Autodesk Inventor part; units mm, degrees
ref_plane "YZ Plane" through (0, 0, 0) normal (1, 0, 0) x (0, 1, 0)
ref_plane "XZ Plane" through (0, 0, 0) normal (0, 1, 0) x (-1, 0, 0)
ref_plane "XY Plane" through (0, 0, 0) normal (0, 0, 1) x (1, 0, 0)
sketch "Sketch1" plane through (0, 0, 0) normal (0, 1, 0) x (-1, 0, 0)
  line L0 (7.4919, 7.8851) -> (-12.5081, 7.8851)
  line L1 (-12.5081, 7.8851) -> (-12.5081, -12.1149)
  line L2 (-12.5081, -12.1149) -> (7.4919, -12.1149)
  line L3 (7.4919, -12.1149) -> (7.4919, 7.8851)
  line L4 (8.4919, 8.8851) -> (-13.5081, 8.8851)
  line L5 (-13.5081, 8.8851) -> (-13.5081, -13.1149)
  line L6 (-13.5081, -13.1149) -> (8.4919, -13.1149)
  line L7 (8.4919, -13.1149) -> (8.4919, 8.8851)
  point P0 (0, 0)
  dimension "d0" = 20
  dimension "d1" = 20
  dimension "d2" = 22
  dimension "d3" = 22
  dimension "d4" = 1
  dimension "d5" = 1
extrude "Extrusion1" add sketch "Sketch1" along normal blind 10 contours L3 L2 L1 L0 | L7 L6 L5 L4
sketch "Sketch2" plane through (0, 0, 0) normal (0, 1, 0) x (-1, 0, 0)
  line L0 (7.4919, 7.8851) -> (-12.5081, 7.8851)
  line L1 (-12.5081, 7.8851) -> (-12.5081, -12.1149)
  line L2 (-12.5081, -12.1149) -> (7.4919, -12.1149)
  line L3 (7.4919, -12.1149) -> (7.4919, 7.8851)
  line L4 (8.4919, -13.1149) -> (8.4919, 8.8851)
  line L5 (8.4919, 8.8851) -> (-13.5081, 8.8851)
  point P0 (0, 0)
  dimension "d8" = 20
  dimension "d9" = 20
  dimension "d10" = 1
  dimension "d11" = 1
extrude "Extrusion2" cut sketch "Sketch2" along normal blind 9
fillet "Fillet1" radius 2 4 edges at (-8.4919, 5, 8.8851) (-8.4919, 5, -13.1149) (13.5081, 5, -13.1149) (13.5081, 5, 8.8851)
properties part number "box"
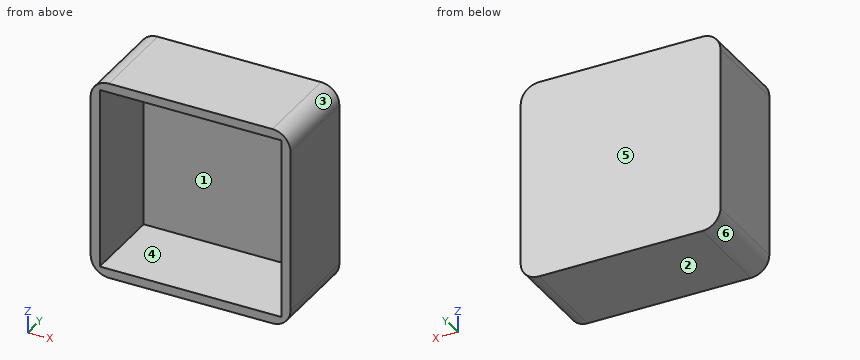
Work out the finished part from the listing and answer in its coordinate system (mm). Face numbers are marked on the shaded views. A direction names the side the tool comes from. Round coordinates to 2 decimals unless told otherwise and drop trailing zeros. Write each loop counter-clockwise with the first axis right and the second up, starting at its lowest first coordinate (ties: lowest second). Pieces come first, ordered by that corner, then holes.
1) A tool of negligible diameter and unlimited length cuts with its end or side. For the marked faces 1 and 2, from which of +Z, -Z, +X, -X, +Y, -Y can it reach the whole face along a straight path? Write none if from no direction.
2) The mould has two halves that part along Z. Classify the marked faces 3, 4, 5 and 6: pulls with the +Z half, pulls with the -Z half, needs draft (parallel to the pull), parting line crosses it, or undercut.
3) A cutting plane is placed at C-C (x = 1.5). Give the vertices of the cut face in (y, z), plus the area to 3 significant figures.
4) Given pin 1 Ø1 at (x, z) = (-2.5, 5.5) entering from -Y, flat-ended and moving along its own axis, determine where the tip first touches the part or whether it passes through.
5) A cutting plane is placed at B-B (z = 5.5). Give the vertices of the cut face in (x, y), plus the area to 3 significant figures.
6) Straight lines are drawn through the part: line 1 (X direction, y = 2, z = -4); line 2 (Z direction, x = 7, y = 2.5); line 3 (Y direction, x = 6.75, z = 1.75). For each, find the intervals that lie inside material, in ascending order.
7) A cutting plane is placed at A-A (y = 6.25). Give the vertices of the cut face in (x, z).
Completed:
1. face 1: -Y
1. face 2: -Z, +X, -X, +Y, -Y
2. face 3: pulls with the +Z half
2. face 4: undercut
2. face 5: needs draft
2. face 6: pulls with the -Z half
3. outline: (0, -13.11) - (10, -13.11) - (10, 8.89) - (0, 8.89) - (0, 7.89) - (9, 7.89) - (9, -12.11) - (0, -12.11) - close
3. area: 40.0 mm2
4. pin 1: stops at y = 9
5. outline: (-8.49, 0) - (-7.49, 0) - (-7.49, 9) - (12.51, 9) - (12.51, 0) - (13.51, 0) - (13.51, 10) - (-8.49, 10) - close
5. area: 40.0 mm2
6. line 1: x = -8.49 to -7.49, 12.51 to 13.51
6. line 2: z = -13.11 to -12.11, 7.89 to 8.89
6. line 3: y = 9 to 10
7. outline: (-8.49, -11.11) arc R2 ccw to (-6.49, -13.11) - (11.51, -13.11) arc R2 ccw to (13.51, -11.11) - (13.51, 6.89) arc R2 ccw to (11.51, 8.89) - (-6.49, 8.89) arc R2 ccw to (-8.49, 6.89) - close; hole (-7.49, -12.11) - (12.51, -12.11) - (12.51, 7.89) - (-7.49, 7.89) - close
